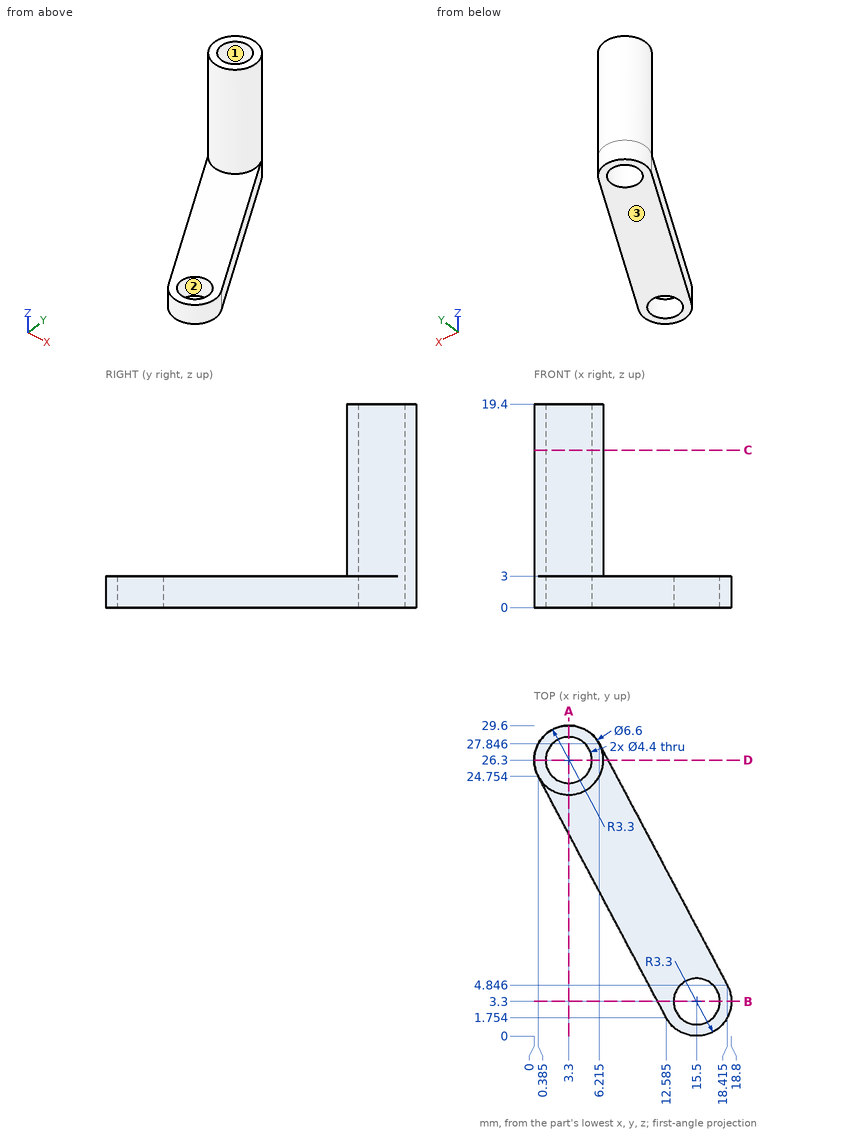
Source: three-view drawing plus pictorial views. Frame: mm from the lowest corner of the part. Give positions to 0.01 mm unless a question says otherwise; leave off trailing zeros. Loops run counter-clockwise (first coordinate to the right, second up) from the corner with the lowest first, then second, coordinate; pieces in that order, holes last. Notation, with made-up numbers: (55, 34) -> (73, 34) arc R24 cw to (73, 49) -> close; hole circle Ø3 at (-28, 20). An arc over 180 degrees is marked (long way). Put each result on its own line as item: value. Start each with the question number.
1) Cut plane C-C (z = 15). Return loops of the section in (x, y) (1 decimal).
2) Cut plane D-D (y = 26.3). Return loops of the section in (x, z) (1 decimal).
3) Cut plane A-A (x = 3.3). Return loops of the section in (y, z).
4) Material intervals for probe 1 along Y at (x, z) = (3.3, 10.25); probe 2 along Z at (x, y) = (7, 23); probe 3 along X at (y, z) = (4, 1) (1 decimal), sorted ascending.
5) Draft query along Y for the marked faces 1, 2 and 3. Return one class per face: released by +Y, released by -Y, zero draft, split by the parting line, or undercut.
6) Contact query for flat-ended pins moving along their axis: P1, Ø6, axis at y = 21.5, z = 11.5, coming from the +X side (1 decimal); P2, Ø8, axis at x = 8, z = 14, coming from the +Y side (1 decimal); P3, Ø1, axis at x = 8, z = 6.5, coming from the +Y side; P4, Ø6, axis at x = 10.5, z = 4.5, coming from the +Y side (1 decimal). Output: stop coordinate, or through.
7) Cut plane B-B (y = 3.3). Return loops of the section in (x, z) (1 decimal).
Results are:
1. outline: circle Ø6.6 at (3.3, 26.3); hole circle Ø4.4 at (3.3, 26.3)
2. outline: (0, 0) -> (1.1, 0) -> (1.1, 19.4) -> (0, 19.4) -> close; (5.5, 0) -> (7, 0) -> (7, 3) -> (6.6, 3) -> (6.6, 19.4) -> (5.5, 19.4) -> close
3. outline: (19.26, 0) -> (24.1, 0) -> (24.1, 19.4) -> (23, 19.4) -> (23, 3) -> (19.26, 3) -> close; (28.5, 0) -> (29.6, 0) -> (29.6, 19.4) -> (28.5, 19.4) -> close
4. probe 1: y = 23 to 24.1, 28.5 to 29.6
4. probe 2: z = 0 to 3
4. probe 3: x = 11.4 to 13.4, 17.6 to 18.7
5. face 1: undercut
5. face 2: undercut
5. face 3: zero draft
6. P1: stops at x = 6.1
6. P2: stops at y = 29.5
6. P3: passes through
6. P4: stops at y = 24.7
7. outline: (11.8, 0) -> (13.3, 0) -> (13.3, 3) -> (11.8, 3) -> close; (17.7, 0) -> (18.8, 0) -> (18.8, 3) -> (17.7, 3) -> close
